Verification items for the finished model (mm, model axes). A direction names the side the tool comes from. Round coordinates to 2 decimals unless told otherwise and drop trailing zeros. Order: outer loops, then holes, each group sorted by start corner. A loop starts at its lowest first (then second) coordinate and runs counter-clockwise, first axis right, second up. Notation, with made-up numbers: (19, 16) -> (74, 16) arc R22 ccw to (74, 23) -> close; hole circle Ø11 at (25.5, -19.5). An arc over 180 degrees is marked (long way). Return JSON: item names as keys, results as strings. Group by question number.
1) Scan lines: L1, parallel to Z at x = 12.5, y = -13; L2, parallel to X at y = 0, z = 20 (3 decimals); L3, parallel to Z at x = 7, y = -11.25 (3 decimals). Record each from-to range of solid material in increasing order.
2) Draft check along Y on faces 1 (the flat face through (0, -14.605, 13)), 2 (the flat face through (-13.335, -13, 18)), 3 (the flat face through (1, -11, 1.905)). Enter one of: pulls with the +Y half, pulls with the -Y half, needs draft (parallel to the pull), parting line crosses it, or undercut.
3) Section check C-C on y = -6.5. Enter the section's corners in (x, z).
4) Depth check by flat-ended pin: pin 1 (1.5 mm diameter, centred on y = -1, z = 21, fed in from +X); pin 2 (4 mm diameter, centred on y = 8, z = 10.5, fed in from +X); pin 3 (1 mm diameter, centred on x = -3.5, y = -8, fed in from +Z); pin 4 (1 mm diameter, centred on y = -4, z = 11, fed in from +X). Enter the tip coordinate at first touch or a pass-through.
5) Section check B-B on y = 7. Enter the section's corners in (x, z), plus the area to 3 significant figures.
6) Tool access check on faces 4 (the flat face through (0, -11, 6.985)), 5 (the flat face through (-10.16, -13, 18)), 6 (the flat face through (-13.335, -13, 7)), 7 (the flat face through (0, -10.478, 4)), 8 (the flat face through (0, -10, 25.4)). Record the directions out of +Z, -Z, +X, -X, +Y, -Y that give a thin tool (end or side, any length) a straight path to the whole face; none if there is none.
7) Section check A-A on x = 0. Enter the section's corners in (y, z) (1 decimal).
8) Section check D-D on x = 4.5. Enter the section's corners in (y, z) (1 decimal).
```python
from build123d import *

# Parameters (mm, degrees)
F1_DEPTH = 25.4
F2_W     = 3.175
F2_H     = 1.5875
F3_DEPTH = 2.566946587
F4_W     = 1.5875
F4_H     = 5.08
F5_DEPTH = 25.4


with BuildPart() as f1:
    # F0 (on Top) → F1 (new body)
    with BuildSketch(Plane.XY):
        with BuildLine():
            ThreePointArc((10.5034451491, -12.065), (8.4074088227, -10.6913747686), (8.8303299626, -8.2212832181))
            ThreePointArc((8.8303299626, -8.2212832181), (4.8153111516, -11.0624140003), (0, -12.065))
            Line((0, -12.065), (10.5034451491, -12.065))
        make_face()
        Polygon((10.5034451491, -12.065), (0, -12.065), (-10.5034451491, -12.065), (-15.875, -12.065), (-15.875, -14.605), (0, -14.605), (15.875, -14.605), (15.875, -12.065), align=None)
        with BuildLine():
            ThreePointArc((0, -12.065), (-4.8153111516, -11.0624140003), (-8.8303299626, -8.2212832181))
            ThreePointArc((-8.8303299626, -8.2212832181), (-8.3761772632, -8.9420248858), (-8.2174451491, -9.779))
            ThreePointArc((-8.2174451491, -9.779), (-8.8869990473, -11.3954461018), (-10.5034451491, -12.065))
            Line((-10.5034451491, -12.065), (0, -12.065))
        make_face()
        with BuildLine():
            ThreePointArc((8.0915303411, 5.0252126064), (9.1596247603, 2.6128335673), (9.525, 0))
            ThreePointArc((9.525, 0), (-2.6128335673, -9.1596247603), (-8.0915303411, 5.0252126064))
            ThreePointArc((-8.0915303411, 5.0252126064), (-7.2937412546, 7.1988383693), (-7.4238053541, 9.5105908894))
            ThreePointArc((-7.4238053541, 9.5105908894), (-7.4818724406, 9.4649780656), (-7.539659283, 9.4190107175))
            ThreePointArc((-7.539659283, 9.4190107175), (-9.0245693038, 8.0075822743), (-10.2492717654, 6.3652693014))
            ThreePointArc((-10.2492717654, 6.3652693014), (-12.0083170813, -1.1681377807), (-8.8303299626, -8.2212832181))
            ThreePointArc((-8.8303299626, -8.2212832181), (-4.8153111516, -11.0624140003), (0, -12.065))
            ThreePointArc((0, -12.065), (4.8153111516, -11.0624140003), (8.8303299626, -8.2212832181))
            ThreePointArc((8.8303299626, -8.2212832181), (11.2272471247, -4.4173687871), (12.065, 0))
            ThreePointArc((12.065, 0), (11.602191363, 3.3095891853), (10.2492717654, 6.3652693014))
            ThreePointArc((10.2492717654, 6.3652693014), (9.0245693038, 8.0075822743), (7.539659283, 9.4190107175))
            ThreePointArc((7.539659283, 9.4190107175), (7.4818724406, 9.4649780656), (7.4238053541, 9.5105908894))
            ThreePointArc((7.4238053541, 9.5105908894), (7.2937412546, 7.1988383693), (8.0915303411, 5.0252126064))
        make_face()
        with BuildLine():
            ThreePointArc((7.6063568635, 10.0761804943), (7.5295347203, 9.7520078104), (7.539659283, 9.4190107175))
            ThreePointArc((7.539659283, 9.4190107175), (9.0245693038, 8.0075822743), (10.2492717654, 6.3652693014))
            ThreePointArc((10.2492717654, 6.3652693014), (9.7859952946, 7.736761108), (9.9797309445, 9.1713625725))
            ThreePointArc((9.9797309445, 9.1713625725), (9.2454528649, 10.8104585739), (7.6063568635, 10.0761804943))
        make_face()
        with BuildLine():
            ThreePointArc((-10.2492717654, 6.3652693014), (-9.0245693038, 8.0075822743), (-7.539659283, 9.4190107175))
            ThreePointArc((-7.539659283, 9.4190107175), (-7.5295347203, 9.7520078104), (-7.6063568635, 10.0761804943))
            ThreePointArc((-7.6063568635, 10.0761804943), (-9.2454528649, 10.8104585739), (-9.9797309445, 9.1713625725))
            ThreePointArc((-9.9797309445, 9.1713625725), (-9.7859952946, 7.736761108), (-10.2492717654, 6.3652693014))
        make_face()
    extrude(amount=F1_DEPTH)

    # F2 (on face) → F3 (cut, through all)
    with BuildSketch(Plane.XZ.offset(14.605)):
        with Locations((-11.7475, 18.25625)):
            Rectangle(F2_W, F2_H)
        with Locations((11.7475, 18.25625)):
            Rectangle(F2_W, F2_H)
        with Locations((11.7475, 7.14375)):
            Rectangle(F2_W, F2_H)
        with Locations((-11.7475, 7.14375)):
            Rectangle(F2_W, F2_H)
    extrude(amount=-F3_DEPTH, mode=Mode.SUBTRACT)

    # F4 (on face) → F5 (cut)
    with BuildSketch(Plane.YZ.offset(15.875)):
        with Locations((-11.27125, 4.445)):
            Rectangle(F4_W, F4_H)
        with Locations((-11.27125, 20.955)):
            Rectangle(F4_W, F4_H)
    extrude(amount=-F5_DEPTH, mode=Mode.SUBTRACT)


solid = f1.part
```
Check result:
{
 "1": {"L1": "0 to 6.35, 7.94 to 17.46, 19.05 to 25.4", "L2": "-12.065 to -9.525, 9.525 to 12.065", "L3": "0 to 1.905, 6.985 to 18.415, 23.495 to 25.4"},
 "2": {"face 1": "pulls with the -Y half", "face 2": "needs draft", "face 3": "undercut"},
 "3": {"outline": "(-10.16, 0) -> (-6.96, 0) -> (-6.96, 25.4) -> (-10.16, 25.4) -> close; (6.96, 0) -> (10.16, 0) -> (10.16, 25.4) -> (6.96, 25.4) -> close"},
 "4": {"pin 1": "x = 12.06", "pin 2": "x = 10.47", "pin 3": "through", "pin 4": "x = 11.55"},
 "5": {"outline": "(-9.95, 0) -> (-7.33, 0) -> (-7.33, 25.4) -> (-9.95, 25.4) -> close; (7.33, 0) -> (9.95, 0) -> (9.95, 25.4) -> (7.33, 25.4) -> close", "area": "133 mm^2"},
 "6": {"face 4": "+X", "face 5": "-Y", "face 6": "+Y, -Y", "face 7": "+X, -X", "face 8": "+Z, +X, -X, +Y, -Y"},
 "7": {"outline": "(-14.6, 0) -> (-9.5, 0) -> (-9.5, 25.4) -> (-14.6, 25.4) -> close; hole (-12.1, 1.9) -> (-10.5, 1.9) -> (-10.5, 7) -> (-12.1, 7) -> close; hole (-12.1, 18.4) -> (-10.5, 18.4) -> (-10.5, 23.5) -> (-12.1, 23.5) -> close"},
 "8": {"outline": "(-14.6, 0) -> (-8.4, 0) -> (-8.4, 25.4) -> (-14.6, 25.4) -> close; hole (-12.1, 1.9) -> (-10.5, 1.9) -> (-10.5, 7) -> (-12.1, 7) -> close; hole (-12.1, 18.4) -> (-10.5, 18.4) -> (-10.5, 23.5) -> (-12.1, 23.5) -> close"}
}
